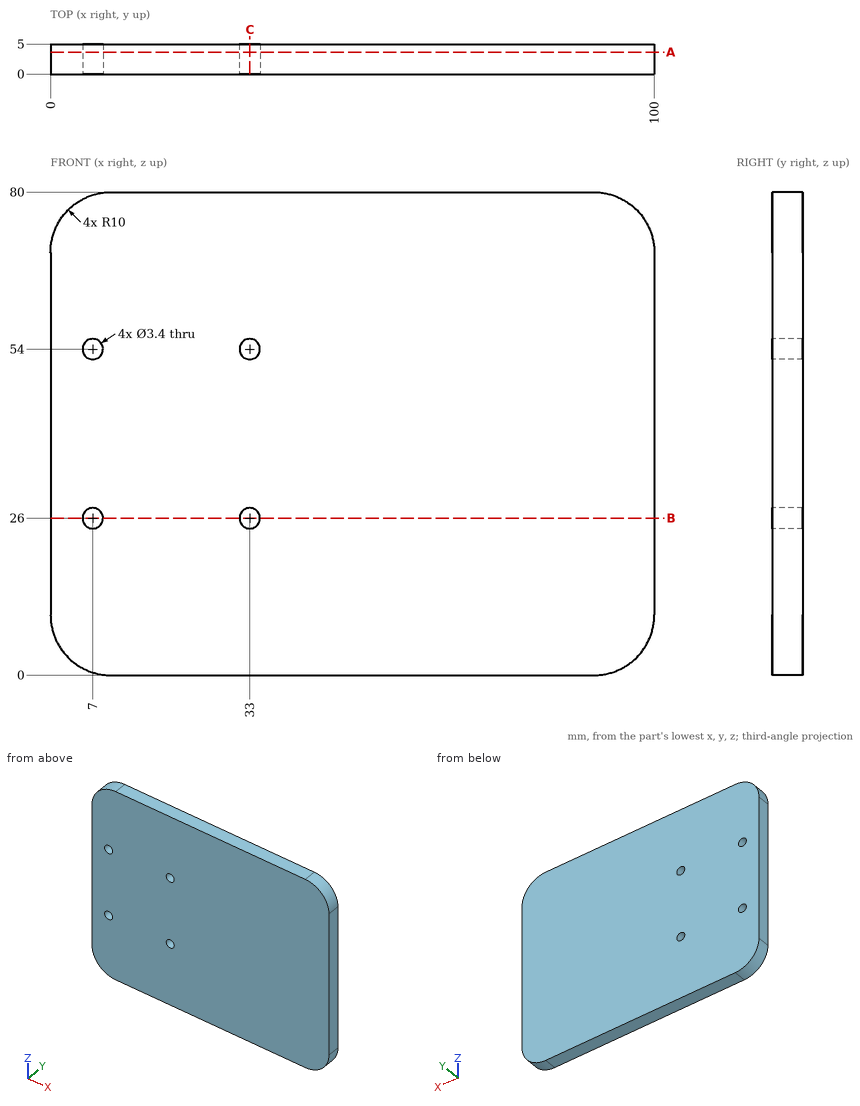
Geometry: see drawing. Coordinates: mm, zero at the bounding-box minimum. Give positions to 0.01 mm unless a question says otherwise; leave off trailing zeros. Write each loop counter-clockwise with the first axis right and the second up, starting at its lowest first coordinate (ties: lowest second). Pieces come first, ordered by that corner, then holes. Notation, with made-up numbers: (-25.75, 47) - (-8.75, 47) arc R27 ccw to (-8.75, 76) - close; hole circle Ø4 at (-39.75, -31). An arc over 180 degrees is marked (long way). Return JSON: item names as keys, results as strings. Group by question number.
1) Section A-A on y = 3.65. Return the cut outline in (x, z).
2) Section C-C on x = 33. Return the cut outline in (y, z), plus the area to 3 significant figures.
3) Section B-B on z = 26. Return the cut outline in (x, y).
4) Line query: line 1 (X direction, y = 3.7, z = 26); line 2 (X direction, y = 2.3, z = 25); line 3 (X direction, y = 3.4, z = 9.5). Output: solid intervals per line, ascending.
Filled in:
{
 "1": {"outline": "(0, 10) arc R10 ccw to (10, 0) - (90, 0) arc R10 ccw to (100, 10) - (100, 70) arc R10 ccw to (90, 80) - (10, 80) arc R10 ccw to (0, 70) - close; hole circle Ø3.4 at (7, 26); hole circle Ø3.4 at (7, 54); hole circle Ø3.4 at (33, 26); hole circle Ø3.4 at (33, 54)"},
 "2": {"outline": "(0, 0) - (5, 0) - (5, 24.3) - (0, 24.3) - close; (0, 27.7) - (5, 27.7) - (5, 52.3) - (0, 52.3) - close; (0, 55.7) - (5, 55.7) - (5, 80) - (0, 80) - close", "area": "366 mm^2"},
 "3": {"outline": "(0, 0) - (5.3, 0) - (5.3, 5) - (0, 5) - close; (8.7, 0) - (31.3, 0) - (31.3, 5) - (8.7, 5) - close; (34.7, 0) - (100, 0) - (100, 5) - (34.7, 5) - close"},
 "4": {"line 1": "x = 0 to 5.3, 8.7 to 31.3, 34.7 to 100", "line 2": "x = 0 to 5.63, 8.37 to 31.63, 34.37 to 100", "line 3": "x = 0.01 to 99.99"}
}
